from build123d import *

# Parameters (mm, degrees)
F0_R     = 2.5
F0_W     = 1625
F0_H     = 550
F1_DEPTH = 5


with BuildPart() as f1:
    # F0 (on Top) → F1 (new body)
    with BuildSketch(Plane.XY):
        Polygon((-749.999512, 52.24733), (-812.499512, -277.75267), (812.500488, -277.75267), (749.994295, 47.936948), align=None)
        with Locations((-167.999512, -267.7244)):
            Circle(F0_R, mode=Mode.SUBTRACT)
        with Locations((-167.999512, -144.441955)):
            Circle(F0_R, mode=Mode.SUBTRACT)
        with Locations((-167.999512, -124.441955)):
            Circle(F0_R, mode=Mode.SUBTRACT)
        with Locations((168.000488, -267.7244)):
            Circle(F0_R, mode=Mode.SUBTRACT)
        with Locations((168.000488, -144.441955)):
            Circle(F0_R, mode=Mode.SUBTRACT)
        with Locations((168.000488, -124.441955)):
            Circle(F0_R, mode=Mode.SUBTRACT)
        with Locations((0.000488, -552.75267)):
            Rectangle(F0_W, F0_H)
        with Locations((-167.999512, -287.7244)):
            Circle(F0_R, mode=Mode.SUBTRACT)
        with Locations((168.000488, -287.7244)):
            Circle(F0_R, mode=Mode.SUBTRACT)
        Polygon((-649.999512, 382.24733), (-749.999512, 52.24733), (749.994295, 47.936948), (649.998543, 384.496444), align=None)
        Polygon((-399.999512, 702.24733), (-649.999512, 382.24733), (649.998543, 384.496444), (400.000488, 702.24733), align=None)
        Polygon((-199.999512, 822.24733), (-399.999512, 702.24733), (400.000488, 702.24733), (200.000486, 822.207413), align=None)
    extrude(amount=-F1_DEPTH)


solid = f1.part
Geometry: final body of the model. Coordinates: model frame, mm. Coordinates: 2 decimals unless noted, no trailing zeros. Order: outer loops, then holes, each group sorted by start corner. A loop starts at its lowest first (then second) coordinate and runs counter-clockwise, first axis right, second up.
1) First-contact query: P1, Ø6.5, axis at x = -168, y = -144.44, coming from the +Z side; P2, Ø3, axis at y = -211, z = -3.5, coming from the -X side; P3, Ø3, axis at y = 55.5, z = -2.5, coming from the +X side. Flat tips, straight axial feed; report the tip coordinate or a pass-through.
Result sheet:
P1: stops at z = 0
P2: stops at x = -800.14
P3: stops at x = 748.19
2) Section C-C (x = 670). Return loops of the section in (y, z).
Result sheet:
outline: (-827.75, -5) - (317.18, -5) - (317.18, 0) - (-827.75, 0) - close
3) Ray query, probe 1 along Y at (x, z) = (-101, -1.25); probe 2 along Y at (x, z) = (588, -4.65); probe 3 along X at (y, z) = (1.5, -1). Return the intervals inside material, ascending.
Result sheet:
probe 1: y = -827.75 to 822.24
probe 2: y = -827.75 to 463.3
probe 3: x = -759.61 to 758.91
4) Section A-A (z = -1.2). Give the number of separate pieces and of enclosed holes in the cut face, then the cut area to 3 significant figures.
Result sheet:
separate pieces: 1
enclosed holes: 8
area: 2,280,000 mm2
5) Section B-B (y = 655.5). Return loops of the section in (x, z), then the cut area to 3 significant figures.
Result sheet:
outline: (-436.52, -5) - (436.78, -5) - (436.78, 0) - (-436.52, 0) - close
area: 4,370 mm2
